```python
from build123d import *

# Parameters (mm, degrees)
SKETCH_R           = 3.5
PAD_DEPTH          = 2
SKETCH001_W        = 4
SKETCH001_H        = 3
PAD001_DEPTH       = 10
POLARPATTERN_COUNT = 4
PAD002_DEPTH       = 10
PAD004_DEPTH       = 2
PAD005_DEPTH       = 20


with BuildPart() as part:
    # Sketch → Pad (new body)
    with BuildSketch(Plane.XY):
        Polygon((-9.8, 2), (-9.8, -2), (-2, -9.8), (2, -9.8), (9.8, -2), (9.8, 2), (2, 9.8), (-2, 9.8), align=None)
        Circle(SKETCH_R, mode=Mode.SUBTRACT)
    extrude(amount=-PAD_DEPTH)

    # Sketch001 → Pad001 (join)
    with BuildSketch(Plane.XY):
        with Locations((0, 8.3)):
            Rectangle(SKETCH001_W, SKETCH001_H)
    pad001 = extrude(amount=PAD001_DEPTH)

    # PolarPattern: Pad001 ×4 about axis
    polarpattern_axis = Axis((0, 0, 0), (0, 0, 1))
    for i in range(1, POLARPATTERN_COUNT):
        add(pad001.rotate(polarpattern_axis, i * 360 / POLARPATTERN_COUNT))

    # Sketch002 → Pad002 (join)
    with BuildSketch(Plane.XY):
        Polygon((-2, 9.8), (-5, 49.8), (5, 49.8), (2, 9.8), align=None)
    extrude(amount=PAD002_DEPTH)

    # Sketch002 → Pad004 (join)
    with BuildSketch(Plane.XY):
        Polygon((-2, 9.8), (-5, 49.8), (5, 49.8), (2, 9.8), align=None)
    extrude(amount=-PAD004_DEPTH)

    # Sketch003 → Pad005 (join, symmetric)
    with BuildSketch(Plane.YZ):
        Polygon((47.684076, 10), (92.389384, 10), (92.389384, 6), (52.389384, 6), (56.797559, -19), (52.797559, -19), align=None)
    extrude(amount=PAD005_DEPTH, both=True)


solid = part.part
```
Can you work these out from the model? Positions are in its coordinate system, mm. A direction names the side the tool comes from. Coordinates: 2 decimals unless noted, no trailing zeros. Order: outer loops, then holes, each group sorted by start corner. A loop starts at its lowest first (then second) coordinate and runs counter-clockwise, first axis right, second up. Notation, with made-up numbers: (61, 67.5) -> (115, 67.5) arc R22 cw to (115, 91.5) -> close; hole circle Ø3 at (39.5, -2). An arc over 180 degrees is marked (long way). Write each question's results on one line, items separated by ' | '.
Item 1: I want a section at B-B, the plane x = 0. Write out the boundary of the cut face in (y, z).
Results are:
outline: (-9.8, -2) -> (-3.5, -2) -> (-3.5, 0) -> (-6.8, 0) -> (-6.8, 10) -> (-9.8, 10) -> close; (3.5, -2) -> (49.8, -2) -> (52.8, -19) -> (56.8, -19) -> (52.39, 6) -> (92.39, 6) -> (92.39, 10) -> (6.8, 10) -> (6.8, 0) -> (3.5, 0) -> close
Item 2: I want a section at D-D, the plane x = -15.5. Write out the boundary of the cut face in (y, z), then the cut area to 3 significant figures.
Results are:
outline: (47.68, 10) -> (52.8, -19) -> (56.8, -19) -> (52.39, 6) -> (92.39, 6) -> (92.39, 10) -> close | area: 277 mm²
Item 3: I'm going to push flat-ended pins straight in: pin 1 Ø1 at (x, y) = (16, 58) entering from -Z; pin 2 Ø2 at (x, z) = (0.5, 4) entering from +Y; pin 3 Ø5 at (x, y) = (-2, 21.5) entering from -Z; pin 4 Ø5 at (x, z) = (-1.5, 4) entering from +Y. Where does each tip first touch, or does it pass through?
Results are:
pin 1: z = 6 | pin 2: y = 52.92 | pin 3: z = -2 | pin 4: y = 92.39
Item 4: If we mould it in two halves opening along Y, with no side actions, what happens to faces 5 (the face through (6.8, 0, 5)), 6 (the face through (8, -2, 5)), 7 (the face through (-8, 2, 5))? For each: +Y half, -Y half, draft (parallel to the pull), parting line (faces both ways), or undercut.
Results are:
face 5: draft | face 6: -Y half | face 7: undercut
Item 5: If I drill on line 1 along Y through (x, z) = (-1, 8.5); line 2 along X through (y, z) = (-1, 1.5); line 3 along Z through (x, y) = (16.5, 81.5), over which ranges is the centre line in solid material (lowest first)?
Results are:
line 1: -9.8 to -6.8, 6.8 to 92.39 | line 2: -9.8 to -6.8, 6.8 to 9.8 | line 3: 6 to 10
Item 6: I want a section at A-A, the plane y = 0. Write out the boundary of the cut face in (x, z), then the cut area to 3 significant figures.
Results are:
outline: (-9.8, -2) -> (-3.5, -2) -> (-3.5, 0) -> (-6.8, 0) -> (-6.8, 10) -> (-9.8, 10) -> close; (3.5, -2) -> (9.8, -2) -> (9.8, 10) -> (6.8, 10) -> (6.8, 0) -> (3.5, 0) -> close | area: 85.2 mm²
Item 7: Which directions (+Z, -Z, +X, -X, +Y, -Y) give clear straight access to the entire face, cutting with the end or side of a thin tool? Please do faces 1 (the face through (2, 8, 5)), 2 (the face through (-2, -8, 5)), 3 (the face through (9.8, 0, 4)), 4 (the face through (0, -6.8, 5)).
Results are:
face 1: +Z, +X, -Y | face 2: +Z, -X, -Y | face 3: +Z, -Z, +X, -Y | face 4: +Z, +X, -X
Item 8: I want a section at C-C, the plane z = 1.25. Write out the boundary of the cut face in (x, y), then the cut area to 3 significant figures.
Results are:
outline: (-20, 49.23) -> (-4.96, 49.23) -> (-2, 9.8) -> (-2, 6.8) -> (2, 6.8) -> (2, 9.8) -> (4.96, 49.23) -> (20, 49.23) -> (20, 53.23) -> (-20, 53.23) -> close; (-9.8, -2) -> (-6.8, -2) -> (-6.8, 2) -> (-9.8, 2) -> close; (-2, -9.8) -> (2, -9.8) -> (2, -6.8) -> (-2, -6.8) -> close; (6.8, -2) -> (9.8, -2) -> (9.8, 2) -> (6.8, 2) -> close | area: 482 mm²
